from build123d import *

# Parameters (mm, degrees)
SKETCH_1_W      = 5
SKETCH_1_H      = 6
SKETCH_1_W_2    = 6
SKETCH_1_H_2    = 2.2
EXTRUDE_1_DEPTH = 150
FILLET_1_R      = 2
FILLET_2_R      = 1


with BuildPart() as part:
    # 스케치1 → 보스-돌출1 (new body)
    with BuildSketch(Plane.XY):
        Polygon((-4.5, 0), (-3, 0), (-2.5, 0), (-2.5, 6), (-2.5, 11), (-4.5, 11), align=None)
        with Locations((0, 3)):
            Rectangle(SKETCH_1_W, SKETCH_1_H)
        Polygon((2.5, 6), (2.5, 0), (3, 0), (4.5, 0), (4.5, 11), (2.5, 11), align=None)
        with Locations((0, -1.1)):
            Rectangle(SKETCH_1_W_2, SKETCH_1_H_2)
        Polygon((3, -2.2), (-3, -2.2), (-5.5, -2.2), (-5.5, -5.2), (5.5, -5.2), (5.5, -2.2), align=None)
    extrude(amount=EXTRUDE_1_DEPTH)

    # 필렛1
    fillet_1_edges = [part.edges().sort_by_distance(p)[0] for p in [
        (-2.5, 8.5, 0),
        (2.5, 8.5, 0),
        (-2.5, 8.5, 150),
        (2.5, 8.5, 150),
        (0, 6, 0),
        (0, 6, 150),
    ]]
    fillet(fillet_1_edges, radius=FILLET_1_R - 0.0001)  # a hair under: the kernel refuses the full size

    # 필렛2
    fillet_2_edges = [part.edges().sort_by_distance(p)[0] for p in [
        (4.25, -2.2, 0),
        (-4.25, -2.2, 0),
        (-3, -1.1, 0),
        (3, -1.1, 0),
    ]]
    fillet(fillet_2_edges, radius=FILLET_2_R)


solid = part.part
The listing builds one solid part. Answer for the finished solid, in the listing's coordinates (mm). A direction names the side the tool comes from. Coordinates: 2 decimals unless noted, no trailing zeros. Write each loop counter-clockwise with the first axis right and the second up, starting at its lowest first coordinate (ties: lowest second). Pieces come first, ordered by that corner, then holes. Notation, with made-up numbers: (46.25, 12) - (85.25, 12) arc R29 ccw to (85.25, 38) - close; hole circle Ø6 at (-36, -33). An arc over 180 degrees is marked (long way). Answer as CSV lines item,"result".
1. Given P1, Ø6, axis at x = 0, y = 6, coming from the -Z side; P2, Ø2.5, axis at y = 7.5, z = 62.5, coming from the -X side; P3, Ø1.5, axis at y = 4.5, z = 135, coming from the +X side; P4, Ø0.7, axis at y = -1.5, z = 87, coming from the +X side, each flat-ended and moving along its own axis, determine where each tip first touches the part or whether it passes through.
Computed values:
P1,"stops at z = 0"
P2,"stops at x = -4.5"
P3,"stops at x = 4.5"
P4,"stops at x = 3"
2. Find section C-C (z = 83). Give the vertices of the cut face in (x, y), plus the area to 3 significant figures.
Computed values:
outline,"(-5.5, -5.2) - (5.5, -5.2) - (5.5, -2.2) - (3, -2.2) - (3, 0) - (4.5, 0) - (4.5, 11) - (2.5, 11) - (2.5, 6) - (-2.5, 6) - (-2.5, 11) - (-4.5, 11) - (-4.5, 0) - (-3, 0) - (-3, -2.2) - (-5.5, -2.2) - close"
area,"120 mm²"
3. A tool of negligible diameter and unlimited length cuts with its end or side. For faces 1 (the flat face through (-4, -2.2, 74)), 2 (the flat face through (-2.5, 8, 74)), 3 (the flat face through (-4.5, 6, 74)), 4 (the flat face through (4, -2.2, 74)), from which of +Z, -Z, +X, -X, +Y, -Y can it reach the whole face along a straight path? Write none if from no direction.
Computed values:
face 1,"+Z, -Z, -X"
face 2,"+Z, -Z, +Y"
face 3,"+Z, -Z, -X, +Y"
face 4,"+Z, -Z, +X"
4. Find section D-D (y = 2.5). Give the vertices of the cut face in (x, z), plus the area to 3 significant figures.
Computed values:
outline,"(-4.5, 0) - (4.5, 0) - (4.5, 150) - (-4.5, 150) - close"
area,"1,350 mm²"
5. Determine the mould class of faces 5 (the flat face through (4.5, 5, 74)), 6 (the flat face through (0, -5.2, 74)), 7 (the flat face through (0, 6, 74)) for opening direction X: +X half, -X half, draft (parallel to the pull), parting line (faces both ways), or undercut.
Computed values:
face 5,"+X half"
face 6,"draft"
face 7,"undercut"
6. Find section B-B (x = 0.25). Give the vertices of the cut face in (y, z).
Computed values:
outline,"(-5.2, 0) - (4, 0) arc R2 ccw to (6, 2) - (6, 148) arc R2 ccw to (4, 150) - (-5.2, 150) - close"
7. Straight lines are drawn through the part: line 1 (X direction, y = 10.25, z = 110.5); line 2 (X direction, y = 5.25, z = 100); line 3 (Y direction, x = -1, z = 21.5). For each, find the intervals that lie inside material, in ascending order. Write a range as [from, to].
Computed values:
line 1,"x = [-4.5, -2.5], [2.5, 4.5]"
line 2,"x = [-4.5, 4.5]"
line 3,"y = [-5.2, 6]"
